Check sheet for the modelled part. Datum: model origin and axes. Units: mm. Coordinates: 2 decimals unless noted, no trailing zeros. Write each loop counter-clockwise with the first axis right and the second up, starting at its lowest first coordinate (ties: lowest second). Pieces come first, ordered by that corner, then holes. Notation, with made-up numbers: (33, 34) -> (78, 34) arc R5 cw to (78, 41) -> close; hole circle Ø8 at (-28.5, 22.5). An arc over 180 degrees is marked (long way). One line per item, written item: value. Start each with the question number.
1) Sectioned sample at C-C on x = 59.5. Enter the section's corners in (y, z).
2) Scan lines: line 1 along X through (y, z) = (2.75, -0.5); line 2 along Y through (x, z) = (61.5, 6.75); line 3 along X through (y, z) = (3.85, 2.5). Record each from-to range of solid material in increasing order. Write a range as [from, to].
3) Sectioned sample at B-B on y = 3.9. Enter the section's corners in (x, z).
4) Sectioned sample at A-A on z = 0. Enter the section's corners in (x, y).
5) Gauge pin test, flat ends, axial feed: P1, Ø2.5, axis at x = -65, z = 0, coming from the -Y side; P2, Ø2, axis at y = 1, z = -1.5, coming from the +X side; P3, Ø4.5, axis at x = 59.5, z = -9.53, coming from the -Y side. Record the tip position at first contact, or that the pin passes through.
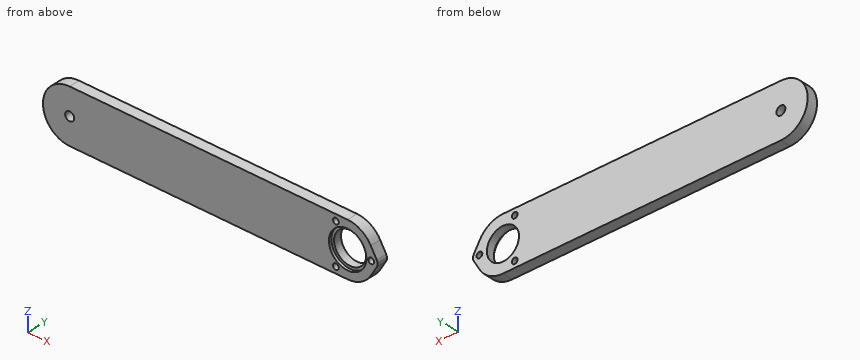
```python
from build123d import *

# Parameters (mm, degrees)
EXTRUDE_1_DEPTH     = 5
EXTRUDE_5_DEPTH     = 5
CUT_EXTRUDE_2_REACH = 82.139
SKETCH_7_R          = 7.5
SKETCH_8_R          = 8.75
CUT_EXTRUDE_3_DEPTH = 1.3
CUT_EXTRUDE_4_REACH = 82.139
SKETCH_9_R          = 1.35
CUT_EXTRUDE_5_REACH = 82.139
SKETCH_12_R         = 2.1


with BuildPart() as part:
    # 草图1 → 凸台-拉伸1 (new body)
    with BuildSketch(Plane(origin=(0, 0, 0), x_dir=(1, 0, 0), z_dir=(0, 1, 0))):
        with BuildLine():
            Line((-65, 12.5), (65, 12.5))
            ThreePointArc((65, 12.5), (77.5, 0), (65, -12.5))
            Line((65, -12.5), (-65, -12.5))
            ThreePointArc((-65, -12.5), (-77.5, 0), (-65, 12.5))
        make_face()
    extrude(amount=EXTRUDE_1_DEPTH)

    # 草图10 → 凸台-拉伸5 (add)
    with BuildSketch(Plane.XZ):
        with BuildLine():
            Line((75.795454545, -6.301441197), (78.590909091, -1.512345887))
            ThreePointArc((78.590909091, -1.512345887), (79, 0), (78.590909091, 1.512345887))
            Line((78.590909091, 1.512345887), (75.795454545, 6.301441197))
            Line((75.795454545, 6.301441197), (75.795454545, -6.301441197))
        make_face()
    extrude(amount=-EXTRUDE_5_DEPTH)

    # 草图7 → 切除-拉伸2 (cut, up to next)
    with BuildSketch(Plane(origin=(0, 5, 0), x_dir=(1, 0, 0), z_dir=(0, 1, 0)), mode=Mode.PRIVATE) as cut_extrude_2_sk1:
        with Locations(Location((65, 0, 0), (0, 0, 270))):
            Circle(SKETCH_7_R)
    cut_extrude_2_tool1 = extrude(cut_extrude_2_sk1.sketch, amount=-CUT_EXTRUDE_2_REACH, mode=Mode.PRIVATE) & part.part
    add(cut_extrude_2_tool1.solids().sort_by_distance((65, 5, 0))[0], mode=Mode.SUBTRACT)

    # 草图8 → 切除-拉伸3 (cut)
    with BuildSketch(Plane(origin=(0, 0, 0), x_dir=(1, 0, 0), z_dir=(0, 1, 0))):
        with Locations(Location((65, 0, 0), (0, 0, 270))):
            Circle(SKETCH_8_R)
    extrude(amount=CUT_EXTRUDE_3_DEPTH, mode=Mode.SUBTRACT)

    # 草图9 → 切除-拉伸4 (cut, up to next)
    with BuildSketch(Plane.XZ, mode=Mode.PRIVATE) as cut_extrude_4_sk1:
        with Locations(Location((59.5, 9.526279442, 0), (0, 0, 270))):
            Circle(SKETCH_9_R)
    cut_extrude_4_tool1 = extrude(cut_extrude_4_sk1.sketch, amount=-CUT_EXTRUDE_4_REACH, mode=Mode.PRIVATE) & part.part
    # 草图9 → 切除-拉伸4 (cut, up to next)
    with BuildSketch(Plane.XZ, mode=Mode.PRIVATE) as cut_extrude_4_sk2:
        with Locations(Location((76, 0, 0), (0, 0, 270))):
            Circle(SKETCH_9_R)
    cut_extrude_4_tool2 = extrude(cut_extrude_4_sk2.sketch, amount=-CUT_EXTRUDE_4_REACH, mode=Mode.PRIVATE) & part.part
    # 草图9 → 切除-拉伸4 (cut, up to next)
    with BuildSketch(Plane.XZ, mode=Mode.PRIVATE) as cut_extrude_4_sk3:
        with Locations(Location((59.5, -9.526279442, 0), (0, 0, 270))):
            Circle(SKETCH_9_R)
    cut_extrude_4_tool3 = extrude(cut_extrude_4_sk3.sketch, amount=-CUT_EXTRUDE_4_REACH, mode=Mode.PRIVATE) & part.part
    add(cut_extrude_4_tool1.solids().sort_by_distance((59.5, 0, 9.526279))[0], mode=Mode.SUBTRACT)
    add(cut_extrude_4_tool2.solids().sort_by_distance((76, 0, 0))[0], mode=Mode.SUBTRACT)
    add(cut_extrude_4_tool3.solids().sort_by_distance((59.5, 0, -9.526279))[0], mode=Mode.SUBTRACT)

    # 草图12 → 切除-拉伸5 (cut, up to next)
    with BuildSketch(Plane(origin=(0, 5, 0), x_dir=(1, 0, 0), z_dir=(0, 1, 0)), mode=Mode.PRIVATE) as cut_extrude_5_sk1:
        with Locations(Location((-65, 0, 0), (0, 0, 270))):
            Circle(SKETCH_12_R)
    cut_extrude_5_tool1 = extrude(cut_extrude_5_sk1.sketch, amount=-CUT_EXTRUDE_5_REACH, mode=Mode.PRIVATE) & part.part
    add(cut_extrude_5_tool1.solids().sort_by_distance((-65, 5, 0))[0], mode=Mode.SUBTRACT)


solid = part.part
```
Answers:
1. outline: (0, -12.5) -> (5, -12.5) -> (5, -10.88) -> (0, -10.88) -> close; (0, -8.18) -> (5, -8.18) -> (5, -5.1) -> (1.3, -5.1) -> (1.3, -6.81) -> (0, -6.81) -> close; (0, 6.81) -> (1.3, 6.81) -> (1.3, 5.1) -> (5, 5.1) -> (5, 8.18) -> (0, 8.18) -> close; (0, 10.88) -> (5, 10.88) -> (5, 12.5) -> (0, 12.5) -> close
2. line 1: x = [-77.49, -67.04], [-62.96, 57.52], [72.48, 74.75], [77.25, 78.96]
2. line 2: y = [1.3, 5]
2. line 3: x = [-77.25, 57.93], [72.07, 78.01]
3. outline: (-65, -12.5) -> (65, -12.5) arc R12.5 ccw to (75.8, -6.3) -> (78.59, -1.51) arc R3 ccw to (78.59, 1.51) -> (75.8, 6.3) arc R12.5 ccw to (65, 12.5) -> (-65, 12.5) arc R12.5 ccw to start; hole circle Ø4.2 at (-65, 0); hole circle Ø15 at (65, 0); hole circle Ø2.7 at (59.5, -9.53); hole circle Ø2.7 at (59.5, 9.53); hole circle Ø2.7 at (76, 0)
4. outline: (-77.5, 0) -> (-67.1, 0) -> (-67.1, 5) -> (-77.5, 5) -> close; (-62.9, 0) -> (56.25, 0) -> (56.25, 1.3) -> (57.5, 1.3) -> (57.5, 5) -> (-62.9, 5) -> close; (72.5, 1.3) -> (73.75, 1.3) -> (73.75, 0) -> (74.65, 0) -> (74.65, 5) -> (72.5, 5) -> close; (77.35, 0) -> (79, 0) -> (79, 5) -> (77.35, 5) -> close
5. P1: passes through
5. P2: stops at x = 78.96
5. P3: stops at y = 0
